Build history of the part. All positions in model axes, mm. A direction names the side the tool comes from. Coordinates: 2 decimals unless noted, no trailing zeros. Loops run counter-clockwise (first coordinate to the right, second up) from the corner with the lowest first, then second, coordinate; pieces in that order, holes last.
Item 1: Cut at B-B (y = -7). List the corners of the cut face in (x, z).
Item 2: Cut at A-A (z = 7.25). List the corners of the cut face in (x, y).
Item 3: Drill centre lines: line 1 along Y through (x, z) = (0, 5.5); line 2 along Y through (x, z) = (-18.5, 12); line 3 along Y through (x, z) = (-8, 10.5). Where is each one in solid material? Low to high.
Item 4: 3-axis set-ups, long thin cutter, end or side, ignore diameter. For faces 1 (the face through (-2.419, 23.794, 3.944)), 2 (the face through (-25, 5, 5)), 3 (the face through (-5.95, -0.05, 2.54)): which of +Z, -Z, +X, -X, +Y, -Y reach the whole face in a straight line?
Item 5: Mould opens along X. For faces 4 (the face through (11, -11, 13.1)), 5 (the face through (-29.97, -1.32, 2.46)), 6 (the face through (5.59, -4.12, 2.54)) say: released by +X, released by -X, zero draft, split by the parting line, or undercut.
Item 6: Cut at D-D (x = 0). Count the separate pieces of the cut face and the enclosed holes in it, and give its area (3 significant figures).
Item 7: Flat gauge pins, fed straight in: pin 1 (5.5 mm diameter, centred on x = 0, y = 20, fed in from -Z); pin 2 (11 mm diameter, centred on x = 0, y = 0, fed in from +Z); pin 3 (1.3 mm diameter, centred on x = 0, y = 7, fed in from -Z); pin 4 (6 mm diameter, centred on x = -20.5, z = 4.5, fed in from -Y). Where does each tip first touch, or does it go through?
Autodesk Inventor part; units mm, degrees
ref_plane "YZ Plane" through (0, 0, 0) normal (1, 0, 0) x (0, 1, 0)
ref_plane "XZ Plane" through (0, 0, 0) normal (0, 1, 0) x (-1, 0, 0)
ref_plane "XY Plane" through (0, 0, 0) normal (0, 0, 1) x (1, 0, 0)
sketch "Sketch1" plane through (0, 0, 0) normal (0, 0, 1) x (1, 0, 0)
  circle A0 centre (0, 0) radius 30
  dimension "d0" = 60
extrude "Extrusion1" add sketch "Sketch1" along normal blind 5
sketch "Sketch2" plane through (0, 0, 5) normal (0, 0, 1) x (1, 0, 0)
  circle A0 centre (0, 0) radius 24.95
  dimension "d3" = 49.9
extrude "Extrusion2" add sketch "Sketch2" along normal blind 8.1
sketch "Sketch3" plane through (0, 0, 13.1) normal (0, 0, 1) x (1, 0, 0)
  circle A0 centre (0, 0) radius 15
  dimension "d6" = 30
extrude "Extrusion3" cut sketch "Sketch3" against normal through all
sketch "Sketch4" plane through (0, 0, 0) normal (0, 0, -1) x (-1, 0, 0)
  circle A0 centre (0, 0) radius 20
  dimension "d9" = 40
extrude "Extrusion4" add sketch "Sketch4" against normal blind 5
sketch "Sketch5" plane through (0, 0, 0) normal (0, 0, -1) x (-1, 0, 0)
  circle A0 centre (0, 0) radius 3.5
  dimension "d12" = 7
extrude "Extrusion5" cut sketch "Sketch5" against normal through all
sketch "Sketch6" plane through (0, 0, 5) normal (0, 0, 1) x (1, 0, 0)
  circle A0 centre (7, 0) radius 1.05
  point P0 (0, 0)
  dimension "d15" = 2.1
  dimension "d16" = 7
extrude "Extrusion6" cut sketch "Sketch6" against normal through all
pattern_circular "Circular Pattern1" count 8 over 360 about axis through (0, 0, -10) along (0, 0, 1) of "Extrusion6"
sketch "Sketch7" plane through (0, 0, 13.1) normal (0, 0, 1) x (1, 0, 0)
  circle A0 centre (-20, 0) radius 2.05
  point P0 (0, 0)
  dimension "d22" = 4.1
  dimension "d23" = 20
extrude "Extrusion7" cut sketch "Sketch7" against normal through all
pattern_circular "Circular Pattern2" count 4 over 360 about axis through (0, 0, -10) along (0, 0, 1) of "Extrusion7"
sketch "Sketch8" plane through (0, 0, 0) normal (0, 0, -1) x (-1, 0, 0)
  circle A0 centre (0, -20) radius 2.05
  circle A1 centre (20, 0) radius 2.05
  circle A2 centre (0, 20) radius 2.05
  circle A3 centre (-20, 0) radius 2.05
  circle A4 centre (0, -20) radius 4.5
  circle A5 centre (20, 0) radius 4.5
  circle A6 centre (0, 20) radius 4.5
  circle A7 centre (-20, 0) radius 4.5
  point P0 (0, 0)
  dimension "d29" = 9
  dimension "d30" = 9
  dimension "d31" = 9
  dimension "d32" = 9
extrude "Extrusion8" cut sketch "Sketch8" against normal blind 8
properties part number "bearing_bracket3"
Filled sheet:
1. outline: (-29.17, 0) - (-1.05, 0) - (-1.05, 5) - (-13.27, 5) - (-13.27, 13.1) - (-23.95, 13.1) - (-23.95, 5) - (-29.17, 5) - close; (1.05, 0) - (29.17, 0) - (29.17, 5) - (23.95, 5) - (23.95, 13.1) - (13.27, 13.1) - (13.27, 5) - (1.05, 5) - close
2. outline: circle Ø49.9 at (0, 0); hole circle Ø9 at (-20, 0); hole circle Ø30 at (0, 0); hole circle Ø9 at (0, -20); hole circle Ø9 at (0, 20); hole circle Ø9 at (20, 0)
3. line 1: y = -24.95 to -24.5, -15.5 to -15, 15 to 15.5, 24.5 to 24.95
3. line 2: y = -16.74 to -1.4, 1.4 to 16.74
3. line 3: y = -23.63 to -12.69, 12.69 to 23.63
4. face 1: -Z
4. face 2: +Z
4. face 3: +Z, -Z
5. face 4: zero draft
5. face 5: split by the parting line
5. face 6: undercut
6. separate pieces: 6
6. enclosed holes: 0
6. area: 219 mm2
7. pin 1: stops at z = 8
7. pin 2: stops at z = 5
7. pin 3: passes through
7. pin 4: stops at y = -24.37
